Geometry check sheet. Reference: the model listing, model coordinates, mm. Face numbers are marked on the shaded views. Coordinates: 2 decimals unless noted, no trailing zeros. Loops run counter-clockwise (first coordinate to the right, second up) from the corner with the lowest first, then second, coordinate; pieces in that order, holes last. Notation, with made-up numbers: (-3.75, 39.5) - (12.25, 39.5) arc R24 cw to (12.25, 70.5) - close; hole circle Ø11 at (-19, 83). An arc over 180 degrees is marked (long way). Write each question's results on one line, items separated by ' | '. Start each with the question number.
(1) Material ranges on probe 1 along Z at (x, y) = (0, -26); probe 2 along X at (y, z) = (-51.5, -2.5); probe 3 along X at (y, z) = (-34, -4.5), recorded low to high.
(2) Go/stop test with a flat-tipped pin: pin 1 Ø2 at (x, z) = (2.5, 3.5) entering from -Y. Record where the tip stops, or that it passes through.
(3) Sectioned sample at C-C (y = 27). Enter the section's corners in (x, z).
(4) Sectioned sample at A-A (x = 0). Enter the section's corners in (y, z).
(5) Mould release check, pull along X, two halves, no side actions. Record for the marked faces 1, 2 and 3: pulls with the +X half, pulls with the -X half, needs draft (parallel to the pull), parting line crosses it, or undercut.
(6) Sectioned sample at B-B (z = 0). Enter the section's corners in (x, y), plus the area to 3 significant figures.
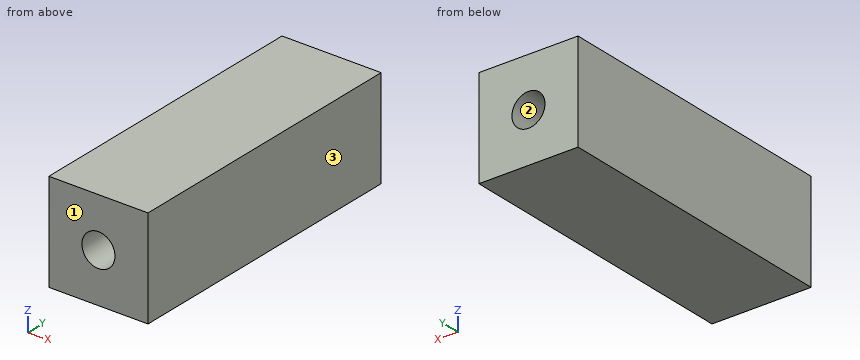
from build123d import *

# Parameters (mm, degrees)
F0_W     = 38.1
F0_H     = 38.1
F1_DEPTH = 57.15
F4_D     = 12.7
F4_DEPTH = 609.6


with BuildPart() as f1:
    # F0 (on Front) → F1 (new body, symmetric)
    with BuildSketch(Plane.XZ):
        Rectangle(F0_W, F0_H)
    extrude(amount=F1_DEPTH, both=True)

    # F4
    with Locations(Plane(origin=(0, 152.4, 0), x_dir=(1, 0, 0), z_dir=(0, 1, 0))):
        with Locations((0, 0)):
            Hole(F4_D / 2, depth=F4_DEPTH)


solid = f1.part
Outcome:
1) probe 1: z = -19.05 to -6.35, 6.35 to 19.05 | probe 2: x = -19.05 to -5.84, 5.84 to 19.05 | probe 3: x = -19.05 to -4.48, 4.48 to 19.05
2) pin 1: passes through
3) outline: (-19.05, -19.05) - (19.05, -19.05) - (19.05, 19.05) - (-19.05, 19.05) - close; hole circle Ø12.7 at (0, 0)
4) outline: (-57.15, -19.05) - (57.15, -19.05) - (57.15, -6.35) - (-57.15, -6.35) - close; (-57.15, 6.35) - (57.15, 6.35) - (57.15, 19.05) - (-57.15, 19.05) - close
5) face 1: needs draft | face 2: undercut | face 3: pulls with the +X half
6) outline: (-19.05, -57.15) - (-6.35, -57.15) - (-6.35, 57.15) - (-19.05, 57.15) - close; (6.35, -57.15) - (19.05, -57.15) - (19.05, 57.15) - (6.35, 57.15) - close | area: 2,900 mm2
